Autodesk Inventor part; units mm, degrees
ref_plane "YZ Plane" through (0, 0, 0) normal (1, 0, 0) x (0, 1, 0)
ref_plane "XZ Plane" through (0, 0, 0) normal (0, 1, 0) x (-1, 0, 0)
ref_plane "XY Plane" through (0, 0, 0) normal (0, 0, 1) x (1, 0, 0)
sketch "スケッチ1" plane through (0, 0, 0) normal (0, 0, 1) x (1, 0, 0)
  line L0 (0, 0) -> (40, 0)
  line L1 (40, 0) -> (40, 318)
  line L2 (40, 318) -> (0, 318)
  line L3 (0, 318) -> (0, 0)
  line L4 (0, 218) -> (112.7627, 152.8964)
  line L5 (112.7627, 152.8964) -> (132.7627, 187.5375)
  line L6 (132.7627, 187.5375) -> (40, 241.094)
  point P0 (40, 218)
  point P1 (40, 194.906)
  point P2 (20, 318)
  point P3 (122.7627, 170.2169)
  point P4 (20, 258)
  dimension "d0" = 40
  dimension "d1" = 318
  dimension "d69" = 40
  dimension "d70" = 60
  dimension "d91" = 20
  dimension "d92" = 100
  dimension "d93" = 180
  dimension "d96" = 20
  dimension "d97" = 60
extrude "押し出し1" add sketch "スケッチ1" along normal blind 19.6 contours L3 L2 L1 L4 | L1 L6 L5 L4
sketch "スケッチ6" plane through (0, 0, 19.6) normal (0, 0, 1) x (1, 0, 0)
  circle A0 centre (20, 268) radius 7
  line L0 (40, 318) -> (0, 318)
  line L1 (40, 241.094) -> (40, 318)
  circle A1 centre (20, 20) radius 1.2295
  circle A2 centre (20, 10) radius 1.2295
  line L2 (0, 0) -> (40, 0)
  circle A3 centre (20, 298) radius 4
  point P0 (20, 318)
  point P1 (40, 190.8114)
  point P2 (30, 0)
  dimension "d42" = 14
  dimension "d44" = 20
  dimension "d45" = 2.459
  dimension "d46" = 2.459
  dimension "d47" = 10
  dimension "d48" = 10
  dimension "d49" = 20
  dimension "d50" = 20
  dimension "d53" = 8
  dimension "d54" = 20
  dimension "d55" = 30
  dimension "d56" = 20
extrude "押し出し4" cut sketch "スケッチ6" against normal through all contours A0 | A3
sketch "スケッチ8" plane through (0, 0, 0) normal (-1, 0, 0) x (0, 0, 1)
  line L0 (0, 318) -> (19.6, 318)
  line L1 (5, 318) -> (14.6, 318)
  line L2 (14.6, 318) -> (14.6, 278)
  line L3 (14.6, 278) -> (5, 278)
  line L4 (5, 278) -> (5, 318)
  line L5 (0, 318) -> (0, 0)
  dimension "d57" = 5
  dimension "d58" = 9.6
  dimension "d59" = 40
  dimension "d98" = 19.6
extrude "押し出し5" cut sketch "スケッチ8" against normal through all
fillet "フィレット1" radius 20 4 edges at (40, 318, 17.1) (40, 318, 2.5) (0, 318, 2.5) (0, 318, 17.1)
fillet "フィレット2" radius 40 2 edges at (0, 218, 9.8) (40, 241.094, 9.8)
sketch "スケッチ9" plane through (0, 0, 19.6) normal (0, 0, 1) x (1, 0, 0)
  line L0 (20, 206.453) -> (112.7627, 152.8964)
  line L1 (132.7627, 187.5375) -> (60, 229.547)
  line L2 (112.7627, 152.8964) -> (132.7627, 187.5375)
  line L3 (132.7627, 187.5375) -> (112.7627, 152.8964)
  line L4 (66.3813, 179.6747) -> (112.7627, 152.8964)
  line L5 (132.7627, 187.5375) -> (166.773, 167.9016)
  line L6 (115.1204, 126.9801) -> (133.5174, 158.8446)
  line L7 (141.7531, 173.1092) -> (128.7627, 180.6092)
  line L8 (112.7627, 152.8964) -> (20, 206.453)
  line L9 (132.7627, 187.5375) -> (60, 229.547)
  line L10 (115.1204, 126.9801) -> (125.7531, 145.3964)
  line L11 (133.5174, 158.8446) -> (145.7531, 180.0375)
  line L12 (116.7627, 159.8246) -> (129.7531, 152.3246)
  line L13 (66.3813, 179.6747) -> (129.7531, 152.3246)
  line L14 (66.3813, 179.6747) -> (86.3813, 214.3157)
  line L15 (86.3813, 214.3157) -> (141.7531, 173.1092)
  point P0 (0, 0)
  point P1 (254.4532, 80.329)
  point P2 (128.7627, 180.6092)
  point P3 (123.2579, 156.0746)
  point P4 (86.3813, 214.3157)
  point P5 (40, 194.906)
  point P6 (115.8875, 158.3088)
  point P7 (129.6379, 182.1251)
  dimension "d80" = 24
  dimension "d81" = 40
  dimension "d83" = 15
  dimension "d84" = 8
  dimension "d90" = 24
extrude "押し出し6" cut sketch "スケッチ9" against normal through all contours L13 L2 L0 | L1 L2 L15
sketch "スケッチ11" plane through (104.9897, 139.4332, 24) normal (0.8660254, -0.5, 0) x (0, 0, -1)
  line L0 (4.4, 21.7957) -> (4.4, 49.2964)
  line L1 (24, 21.7957) -> (24, 49.2964)
  line L2 (0, 24) -> (24, 24)
  line L3 (24, 24) -> (24, 0)
  line L4 (24, 0) -> (0, 0)
  line L5 (0, 0) -> (0, 24)
  line L6 (17, 17) -> (7, 17)
  line L7 (7, 17) -> (7, 7)
  line L8 (7, 7) -> (17, 7)
  line L9 (17, 7) -> (17, 17)
  line L10 (4.4, 35.546) -> (24, 35.546)
  circle A0 centre (14.2, 35.546) radius 5
  point P0 (24, -173.2475)
  point P1 (24, 24)
  point P2 (0, 15.546)
  point P3 (24, 15.546)
  dimension "d85" = 10
  dimension "d88" = 10
extrude "押し出し7" add sketch "スケッチ11" along normal blind 15 contours A0 L10 | L10 A0
fillet "フィレット4" radius 20 2 edges at (0, 278, 9.8) (40, 278, 9.8)
sketch "スケッチ12" plane through (0, 0, 19.6) normal (0, 0, 1) x (1, 0, 0)
  line L0 (0, 340.2847) -> (40, 340.2847)
  line L1 (40, 340.2847) -> (40, 181.2581)
  line L2 (40, 181.2581) -> (0, 181.2581)
  line L3 (0, 181.2581) -> (0, 340.2847)
  line L4 (40, 264.188) -> (40, 298)
  arc A0 (40, 298) -> (0, 298) centre (20, 298) ccw
  arc A1 (40, 264.188) -> (60, 229.547) centre (80, 264.188) ccw
  line L5 (60, 229.547) -> (40, 194.906)
  line L6 (20, 206.453) -> (66.3813, 179.6747)
  arc A2 (0, 241.094) -> (20, 206.453) centre (40, 241.094) ccw
  arc A3 (0, 241.094) -> (20, 206.453) centre (40, 241.094) ccw
  line L7 (20, 206.453) -> (40, 194.906)
  line L8 (86.3813, 214.3157) -> (60, 229.547)
  line L9 (60, 229.547) -> (86.3813, 214.3157)
  line L10 (86.3813, 214.3157) -> (66.3813, 179.6747)
  line L11 (40, 194.906) -> (66.3813, 179.6747)
  circle A4 centre (20, 298) radius 4
  circle A5 centre (20, 268) radius 7
  circle A6 centre (20, 268) radius 4
  point P0 (0, 0)
  dimension "d99" = 40
  dimension "d100" = 40
extrude "押し出し8" add sketch "スケッチ12" along normal blind 5 contours A0 L1 L6 A2 L3 | A1 L5 L1 | L5 L8 L10 L6
sketch "スケッチ13" plane through (0, 0, 0) normal (0, 0, -1) x (-1, 0, 0)
  line L0 (-253.843, 397.4333) -> (123.9074, 397.4333)
  line L1 (123.9074, 397.4333) -> (123.9074, 95.9261)
  line L2 (123.9074, 95.9261) -> (-253.843, 95.9261)
  line L3 (-253.843, 95.9261) -> (-253.843, 397.4333)
  point P0 (0, 0)
extrude "押し出し9" cut sketch "スケッチ13" against normal blind 19.6
sketch "スケッチ14" plane through (0, 0, 24.6) normal (0, 0, 1) x (1, 0, 0)
  line L0 (20, 206.453) -> (66.3813, 179.6747)
  line L1 (66.3813, 179.6747) -> (86.3813, 214.3157)
  line L2 (41.7403, 216.9952) -> (76.3813, 196.9952)
  point P0 (0, 0)
  point P1 (67.7211, 201.9952)
  dimension "d105" = 20
  dimension "d106" = 20
  dimension "d107" = 30
  dimension "d108" = 10
hole "穴3" at (41.7403, 216.9952, 24.6) at (67.7211, 201.9952, 24.6) direction (0, 0, -1) diameter 3 end through all
fillet "フィレット5" radius 5 2 edges at (86.3813, 214.3157, 22.1) (66.3813, 179.6747, 22.1)
sketch "スケッチ15" plane through (0, 0, 24.6) normal (0, 0, 1) x (1, 0, 0)
  circle A0 centre (41.7403, 216.9952) radius 1.5
  circle A1 centre (41.7403, 216.9952) radius 3
  circle A2 centre (67.7211, 201.9952) radius 1.5
  circle A3 centre (67.7211, 201.9952) radius 3
  point P0 (0, 0)
  dimension "d117" = 6
  dimension "d118" = 6
extrude "押し出し10" cut sketch "スケッチ15" against normal blind 3
equation "\"d45\" = d46"
equation "\"d48\" = d47"
equation "\"d50\" = d49"
equation "\"d106\" = d105"
properties part number "BR_parts_06(1)" material "アルミニウム 6061"
Geometry check sheet. Reference: the model listing, model coordinates, mm. A direction names the side the tool comes from. Coordinates: 2 decimals unless noted, no trailing zeros. Order: outer loops, then holes, each group sorted by start corner. A loop starts at its lowest first (then second) coordinate and runs counter-clockwise, first axis right, second up.
Item 1: Mould release check, pull along Y, two halves, no side actions. Record for faces 4 (the flat face through (40, 216, 21.6)), 5 (the flat face through (33, 251, 19.6)), 6 (the cylindrical face through (41.674, 218.494, 20.586)), 7 (the cylindrical face through (84.4, 213.7, 22.1)): released by +Y, released by -Y, zero draft, split by the parting line, or undercut.
Item 2: Section check D-D (x = 49). Enter the section's corners in (y, z).
Item 3: Tool access check on faces 1 (the cylindrical face through (64.724, 202.127, 23.121)), 2 (the flat face through (40, 281, 22)), 3 (the cylindrical face through (20, 318, 22)). Record the directions out of +Z, -Z, +X, -X, +Y, -Y that give a thin tool (end or side, any length) a straight path to the whole face; none if there is none.
Item 4: Scan lines: line 1 along Y through (x, z) = (20, 23); line 2 along X through (y, z) = (268, 22); line 3 along X through (y, z) = (298, 22.85). Record each from-to range of solid material in increasing order.
Item 5: Depth check by flat-ended pin: pin 1 (3.5 mm diameter, centred on x = 67.72, y = 202, fed in from +Z); pin 2 (3 mm diameter, centred on y = 238, z = 22.5, fed in from -X); pin 3 (5 mm diameter, centred on x = 20, y = 298, fed in from -Z); pin 4 (1.5 mm diameter, centred on y = 288, z = 22, fed in from +X). Enter the tip coordinate at first touch or a pass-through.
Item 6: Section check C-C (z = 22.55). Enter the section's corners in (x, y).
Item 7: Section check B-B (x = 14.5). Enter the section's corners in (y, z), plus the area to 3 significant figures.
Item 8: Section check A-A (y = 268). Enter the section's corners in (x, z), plus the area to 3 significant figures.
Check sheet entries:
1. face 4: undercut
1. face 5: zero draft
1. face 6: undercut
1. face 7: split by the parting line
2. outline: (189.71, 19.6) - (238.91, 19.6) - (238.91, 24.6) - (189.71, 24.6) - close
3. face 1: +Z
3. face 2: +Z, -Z, +X, +Y
3. face 3: +Z, -Z, +Y
4. line 1: y = 206.45 to 261, 275 to 294, 302 to 318
4. line 2: x = 0 to 13, 27 to 40
4. line 3: x = 0 to 16, 24 to 40
5. pin 1: stops at z = 21.6
5. pin 2: stops at x = 0.03
5. pin 3: passes through
5. pin 4: stops at x = 40
6. outline: (0, 241.09) arc R40 ccw to (20, 206.45) - (62.05, 182.17) arc R5 ccw to (68.88, 184) - (83.88, 209.99) arc R5 ccw to (82.05, 216.82) - (60, 229.55) arc R40 cw to (40, 264.19) - (40, 298) arc R20 ccw to (0, 298) - close; hole circle Ø14 at (20, 268); hole circle Ø8 at (20, 298); hole circle Ø6 at (41.74, 217); hole circle Ø6 at (67.72, 202)
7. outline: (210.28, 19.6) - (263.67, 19.6) - (263.67, 24.6) - (210.28, 24.6) - close; (272.33, 19.6) - (317.23, 19.6) - (317.23, 24.6) - (272.33, 24.6) - close
7. area: 491 mm2
8. outline: (0, 19.6) - (13, 19.6) - (13, 24.6) - (0, 24.6) - close; (27, 19.6) - (40, 19.6) - (40, 24.6) - (27, 24.6) - close
8. area: 130 mm2
